Geometry: final body of the model. Coordinates: model frame, mm. Coordinates: 2 decimals unless noted, no trailing zeros. Loops run counter-clockwise (first coordinate to the right, second up) from the corner with the lowest first, then second, coordinate; pieces in that order, holes last. Notation, with made-up numbers: (32.5, 38.25) - (36.5, 38.25) arc R21 cw to (36.5, 67.25) - close; hole circle Ø10 at (31.25, 33.5). An arc over 180 degrees is marked (long way). Put each result on its own line as item: value. Start each with the question number.
1) Section A-A on z = 75. Output: boundary loops of the cut face in (x, y).
2) Contact query for flat-ended pins moving along their axis: pin 1 Ø1.5 at (y, z) = (3, -227.5) entering from -X; pin 2 Ø5 at (x, y) = (-211.5, 7.5) entering from +Z; pin 3 Ø1.5 at (y, z) = (6, -116.5) entering from -X. Output: stop coordinate, or through.
3) Section B-B on x = 19.5. Output: boundary loops of the cut face in (y, z) (3 decimals), and give its area (3 significant figures).
4) Section C-C on y = 5.5. Output: boundary loops of the cut face in (x, z).
5) Section D-D on x = -113. Output: boundary loops of the cut face in (y, z), and give its area (3 significant figures).
6) Material intervals for line 1 along Z through (x, y) = (11, 7); line 2 along X through (y, z) = (6.5, 119); line 3 along X through (y, z) = (6.5, 80.5), sorted ascending. Write a range as from..to.
```python
from build123d import *

# Parameters (mm, degrees)
ESQUISSE1_R        = 300
ESQUISSE1_R_2      = 11.902763715
BOSS_EXTRU_1_DEPTH = 10


with BuildPart() as part:
    # Esquisse1 → Boss.-Extru.1 (new body)
    with BuildSketch(Plane(origin=(0, 0, 0), x_dir=(1, 0, 0), z_dir=(0, 1, 0))):
        with Locations(Location((0, 0, 0), (0, 0, 270))):
            Circle(ESQUISSE1_R)
        with Locations(Location((-34.641016151, -130, 0), (0, 0, 270))):
            Circle(ESQUISSE1_R_2, mode=Mode.SUBTRACT)
        with Locations(Location((129.903810568, -75, 0), (0, 0, 270))):
            Circle(ESQUISSE1_R_2, mode=Mode.SUBTRACT)
        with BuildLine():
            Line((-34.641016151, -20), (-5.951381857, 29.691904248))
            ThreePointArc((-5.951381857, 29.691904248), (-5.951381857, 50.308095752), (11.902763715, 40))
            ThreePointArc((11.902763715, 40), (10.308095752, 34.048618143), (5.951381857, 29.691904248))
            Line((5.951381857, 29.691904248), (34.641016151, -20))
            Line((34.641016151, -20), (-34.641016151, -20))
        make_face(mode=Mode.SUBTRACT)
    extrude(amount=BOSS_EXTRU_1_DEPTH)


solid = part.part
```
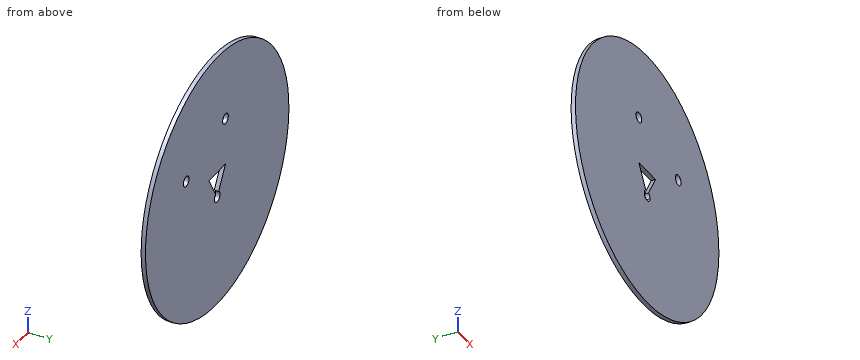
Answer block:
1. outline: (-290.47, 0) - (118, 0) - (118, 10) - (-290.47, 10) - close; (141.81, 0) - (290.47, 0) - (290.47, 10) - (141.81, 10) - close
2. pin 1: stops at x = -196.43
2. pin 2: stops at z = 215.22
2. pin 3: stops at x = -276.77
3. outline: (0, -299.366) - (10, -299.366) - (10, -6.225) - (0, -6.225) - close; (0, 20) - (10, 20) - (10, 299.366) - (0, 299.366) - close
3. area: 5,730 mm²
4. outline: circle Ø600 at (0, 0); hole circle Ø23.81 at (-34.64, 130); hole (-34.64, 20) - (-5.95, -29.69) arc R11.9 ccw (long way) to (5.95, -29.69) - (34.64, 20) - close; hole circle Ø23.81 at (129.9, 75)
5. outline: (0, -277.9) - (10, -277.9) - (10, 277.9) - (0, 277.9) - close
5. area: 5,560 mm²
6. line 1: z = -299.8..-44.55, -35.45..-20.95, 20..299.8
6. line 2: x = -275.39..-39.19, -30.09..275.39
6. line 3: x = -289..119.35, 140.46..289
